```python
from build123d import *

# Parameters (mm, degrees)
SKETCH1_R           = 25
BOSS_EXTRUDE1_DEPTH = 29.7
SKETCH2_R           = 11
BOSS_EXTRUDE2_DEPTH = 6
SKETCH3_R           = 12.25
BOSS_EXTRUDE3_DEPTH = 9
SKETCH4_R           = 3.5
CUT_EXTRUDE1_DEPTH  = 57.992016985


with BuildPart() as part:
    # Sketch1 → Boss-Extrude1 (new body)
    with BuildSketch(Plane.XY):
        Circle(SKETCH1_R)
    extrude(amount=BOSS_EXTRUDE1_DEPTH)

    # Sketch2 → Boss-Extrude2 (add)
    with BuildSketch(Plane.XY.offset(29.7)):
        Circle(SKETCH2_R)
    extrude(amount=BOSS_EXTRUDE2_DEPTH)

    # Sketch3 → Boss-Extrude3 (add)
    with BuildSketch(Plane(origin=(0, 0, 0), x_dir=(-1, 0, 0), z_dir=(0, 0, -1))):
        Circle(SKETCH3_R)
    extrude(amount=BOSS_EXTRUDE3_DEPTH)

    # Sketch4 → Cut-Extrude1 (cut, through all)
    with BuildSketch(Plane(origin=(0, 0, -9), x_dir=(-1, 0, 0), z_dir=(0, 0, -1))):
        Circle(SKETCH4_R)
    extrude(amount=-CUT_EXTRUDE1_DEPTH, mode=Mode.SUBTRACT)


solid = part.part
```
Can you work these out from the model? Positions are in its coordinate system, mm. A direction names the side the tool comes from. Coordinates: 2 decimals unless noted, no trailing zeros. Write each loop counter-clockwise with the first axis right and the second up, starting at its lowest first coordinate (ties: lowest second). Pieces come first, ordered by that corner, then holes. Notation, with made-up numbers: (10, -13) - (50, -13) arc R17 ccw to (50, 4) - close; hole circle Ø6 at (75, 16.5). An arc over 180 degrees is marked (long way). Return JSON: item names as keys, results as strings.
Q1. If we section it at C-C (z = 5): Please give me the cut outline in (x, y), then the cut area to 3 significant figures.
Computed values:
{"outline": "circle Ø50 at (0, 0); hole circle Ø7 at (0, 0)", "area": "1,930 mm2"}
Q2. Thinking about a two-plate mould opening in Y: for faces 4 (the flat face through (-3, 3, 35.7)), 5 (the cylindrical face through (-3.233, -1.341, 13.037)), 6 (the cylindrical face through (-2.38, -10.74, 32.66)), which applies, +Y half, -Y half, draft (parallel to the pull), parting line (faces both ways), or undercut?
Computed values:
{"face 4": "draft", "face 5": "undercut", "face 6": "parting line"}
Q3. Please list where these lines run through material, in increasing order: L1, parallel to Y at x = 0, z = 1.5; L2, parallel to Z at x = 9.5, y = -17; L3, parallel to X at y = 13.5, z = 24. Write a range as from..to.
Computed values:
{"L1": "y = -25..-3.5, 3.5..25", "L2": "z = 0..29.7", "L3": "x = -21.04..21.04"}
Q4. If we section it at A-A (y = 0): Please give me the cut outline in (x, z), then the cut area to 3 significant figures.
Computed values:
{"outline": "(-25, 0) - (-12.25, 0) - (-12.25, -9) - (-3.5, -9) - (-3.5, 35.7) - (-11, 35.7) - (-11, 29.7) - (-25, 29.7) - close; (3.5, -9) - (12.25, -9) - (12.25, 0) - (25, 0) - (25, 29.7) - (11, 29.7) - (11, 35.7) - (3.5, 35.7) - close", "area": "1,520 mm2"}
Q5. I'm going to push flat-ended pins straight in: pin 1 Ø8 at (x, z) = (3.5, -0.5) entering from -Y; pin 2 Ø4 at (y, z) = (10, 15) entering from +X; pin 3 Ø3 at (x, y) = (-18.5, -4) entering from -Z. Where does each tip first touch, or does it pass through?
Computed values:
{"pin 1": "stops at y = -25", "pin 2": "stops at x = 23.69", "pin 3": "stops at z = 0"}
Q6. If we section it at D-D (x = -10): Please give me the cut outline in (y, z).
Computed values:
{"outline": "(-22.91, 0) - (-7.08, 0) - (-7.08, -9) - (7.08, -9) - (7.08, 0) - (22.91, 0) - (22.91, 29.7) - (4.58, 29.7) - (4.58, 35.7) - (-4.58, 35.7) - (-4.58, 29.7) - (-22.91, 29.7) - close"}
Q7. On a 3-axis mill with a long thin cutter (end or side, diameter ignored), from which of +Z, -Z, +X, -X, +Y, -Y can I reach the whole of each face in a straight line? I mean faces 1 (the flat face through (-3, -3, -9)), 2 (the flat face through (-6, -11, 0)), 3 (the flat face through (5, -11, 29.7)). Say none if no direction works.
Computed values:
{"face 1": "-Z, +X, -X, +Y, -Y", "face 2": "-Z", "face 3": "+Z"}
